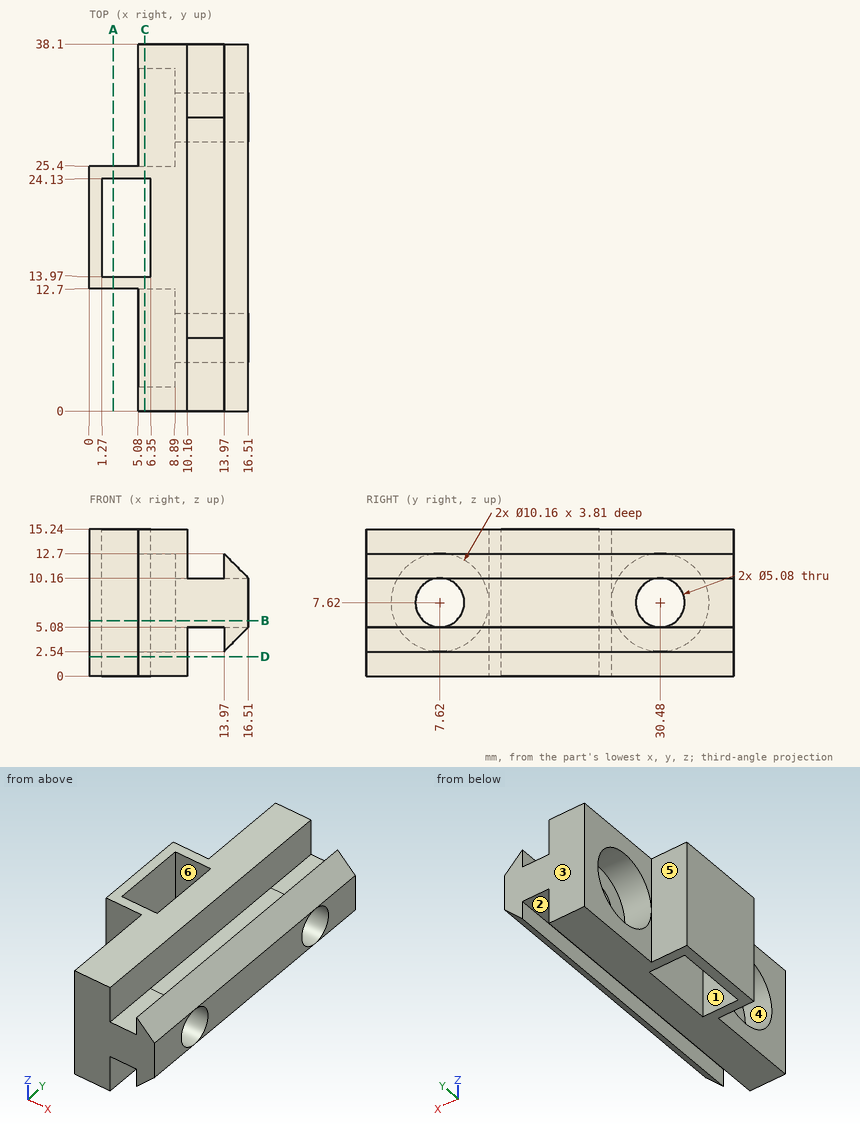
Job drawing, mm, ordinate dimensions from the low corner. One solid piece. A direction names the side the tool comes from. Round coordinates to 2 decimals unless told otherwise and drop trailing zeros. Order: outer loops, then holes, each group sorted by start corner. A loop starts at its lowest first (then second) coordinate and runs counter-clockwise, first axis right, second up. Notation, with made-up numbers: (-31, 4.5) -> (-24, 4.5) arc R25 ccw to (-24, 19.5) -> close; hole circle Ø1 at (88, 21.5). An arc over 180 degrees is marked (long way). Write item = value, one per line.
(1) Flat gauge pins, fed straight in: P1, Ø1.5, axis at y = 23, z = 13, coming from the +X side; P2, Ø0.8, axis at y = 11, z = 4, coming from the -X side; P3, Ø1.9, axis at x = 12, y = 19, coming from the -Z side. Where does each tip first touch, or does it go through?
Answers follow:
P1 = 14.42
P2 = 5.08
P3 = 5.08
(2) Drill centre lines: L1, parallel to Y at x = 5.9, z = 7.62; L2, parallel to Y at x = 8, z = 7.62; L3, parallel to Z at x = 7.35, y = 30.48. Where is each one in solid material? Low to high.
Answers follow:
L1 = 0 to 2.54, 12.7 to 13.97, 24.13 to 25.4, 35.56 to 38.1
L2 = 0 to 2.54, 12.7 to 25.4, 35.56 to 38.1
L3 = 0 to 2.54, 12.7 to 15.24
(3) Cut at C-C (x = 5.75). Write the cut outline in (y, z), plus the area to 3 significant figures.
Answers follow:
outline = (0, 0) -> (13.97, 0) -> (13.97, 15.24) -> (0, 15.24) -> close; (24.13, 0) -> (38.1, 0) -> (38.1, 15.24) -> (24.13, 15.24) -> close; hole circle Ø10.16 at (7.62, 7.62); hole circle Ø10.16 at (30.48, 7.62)
area = 264 mm²
(4) Cut at B-B (z = 5.75). Write the cut outline in (x, y), plus the area to 3 significant figures.
Answers follow:
outline = (0, 12.7) -> (5.08, 12.7) -> (5.08, 12.34) -> (8.89, 12.34) -> (8.89, 9.34) -> (16.51, 9.34) -> (16.51, 28.76) -> (8.89, 28.76) -> (8.89, 25.76) -> (5.08, 25.76) -> (5.08, 25.4) -> (0, 25.4) -> close; (5.08, 0) -> (16.51, 0) -> (16.51, 5.9) -> (8.89, 5.9) -> (8.89, 2.9) -> (5.08, 2.9) -> close; (5.08, 35.2) -> (8.89, 35.2) -> (8.89, 32.2) -> (16.51, 32.2) -> (16.51, 38.1) -> (5.08, 38.1) -> close; hole (1.27, 13.97) -> (6.35, 13.97) -> (6.35, 24.13) -> (1.27, 24.13) -> close
area = 324 mm²
(5) Cut at A-A (x = 2.5). Write the cut outline in (y, z), plus the area to 3 significant figures.
Answers follow:
outline = (12.7, 0) -> (13.97, 0) -> (13.97, 15.24) -> (12.7, 15.24) -> close; (24.13, 0) -> (25.4, 0) -> (25.4, 15.24) -> (24.13, 15.24) -> close
area = 38.7 mm²
(6) 3-axis set-ups, long thin cutter, end or side, ignore diameter. For the marked faces 4, 5 and 6: which of +Z, -Z, +X, -X, +Y, -Y reach the whole face in a straight line?
Answers follow:
face_4 = -X
face_5 = +Z, -Z, -X, +Y
face_6 = +Z, -Z
(7) Pull direction Y, two halves, no side cores. Call the marked faces 1, 2 and 3: +Y half, -Y half, draft (parallel to the pull), parting line (faces both ways), or undercut.
Answers follow:
face_1 = undercut
face_2 = draft
face_3 = +Y half
(8) Cut at D-D (z = 2). Write the cut outline in (x, y).
Answers follow:
outline = (0, 12.7) -> (5.08, 12.7) -> (5.08, 0) -> (10.16, 0) -> (10.16, 38.1) -> (5.08, 38.1) -> (5.08, 25.4) -> (0, 25.4) -> close; hole (1.27, 13.97) -> (6.35, 13.97) -> (6.35, 24.13) -> (1.27, 24.13) -> close
